For this review, use the dimensioned drawing (mm, ordinates from the lowest corner) and the shaded views. Coordinates: 2 decimals unless noted, no trailing zeros. Write each loop counter-clockwise with the first axis right and the second up, starting at its lowest first coordinate (ties: lowest second). Pieces come first, ordered by that corner, then holes. Notation, with made-up numbers: (8, 73.5) - (25, 73.5) arc R17 cw to (25, 101.5) - close; hole circle Ø10 at (16, 78.5). An arc over 180 degrees is marked (long way). One line per item, written item: value.
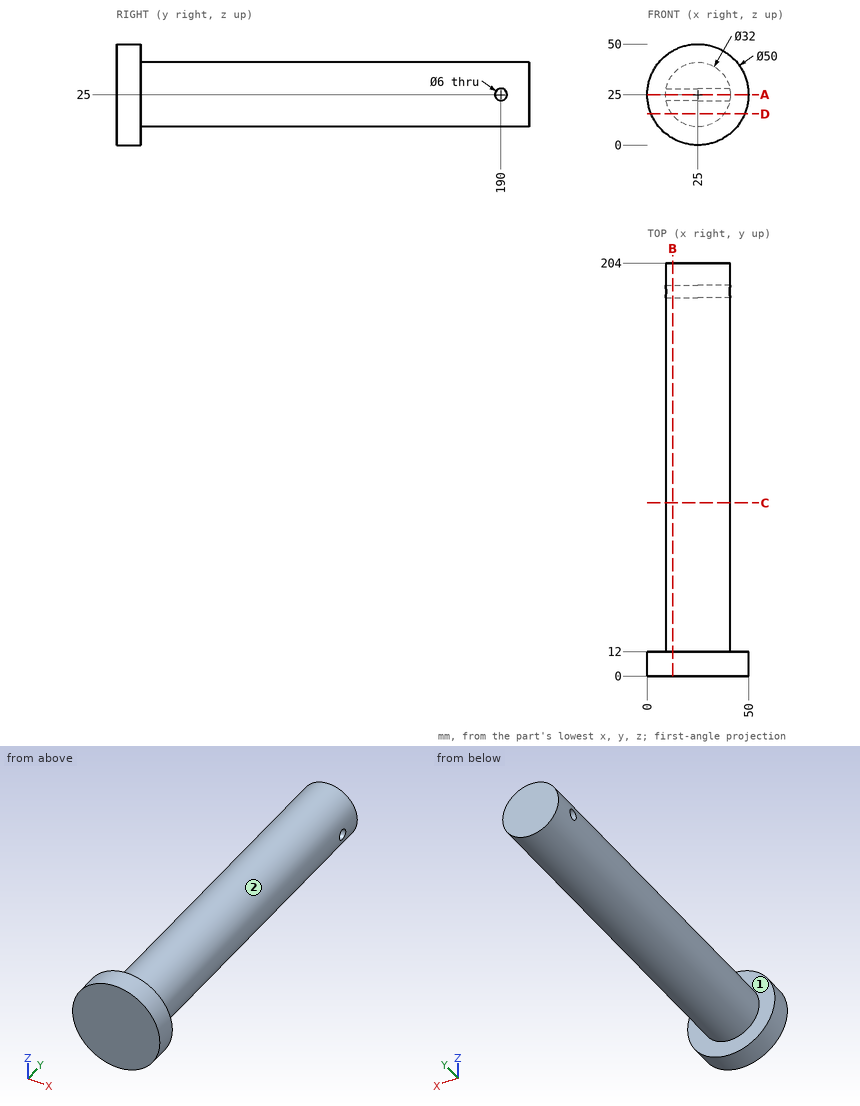
1. Wall thickness on line 1 along Y through (x, z) = (18, 25); line 2 along Y through (x, z) = (22, 43.5); line 3 along Y through (x, z) = (23, 27): over which ranges is each line inside the solid? List them lowest first.
Answer block:
line 1: y = 0 to 187, 193 to 204
line 2: y = 0 to 12
line 3: y = 0 to 187.76, 192.24 to 204
2. Consider section C-C, the plane y = 85.5. Write out the cut boundary in (x, z), then the cut area to 3 significant figures.
Answer block:
outline: circle Ø32 at (25, 25)
area: 804 mm^2
3. Consider section A-A, the plane z = 25. Write out the cut boundary in (x, y), then the cut area to 3 significant figures.
Answer block:
outline: (0, 0) - (50, 0) - (50, 12) - (41, 12) - (41, 187) - (9, 187) - (9, 12) - (0, 12) - close; (9, 193) - (41, 193) - (41, 204) - (9, 204) - close
area: 6,550 mm^2
4. Consider section D-D, the plane z = 15.5. Write out the cut boundary in (x, y).
Answer block:
outline: (1.88, 0) - (48.12, 0) - (48.12, 12) - (37.87, 12) - (37.87, 204) - (12.13, 204) - (12.13, 12) - (1.88, 12) - close
5. Mouldability with a two-part tool opening along X and no side actions: class the marked faces 1 and 2 as released by +X, released by -X, zero draft, split by the parting line, or undercut.
Answer block:
face 1: zero draft
face 2: split by the parting line
6. Insertion check: pin 1 Ø2 at (x, y) = (39, 20.5) entering from +Z; pin 2 Ø12 at (y, z) = (96.5, 39.5) entering from -X; pin 3 Ø8 at (y, z) = (190, 25) entering from -X. Each pin has a flat end and moves straight along its axis. Give the tip position at first contact, or say it passes through.
Answer block:
pin 1: stops at z = 34.33
pin 2: stops at x = 11.44
pin 3: stops at x = 9
7. Consider section B-B, the plane x = 12.5. Write out the cut boundary in (y, z), then the cut area to 3 significant figures.
Answer block:
outline: (0, 3.35) - (12, 3.35) - (12, 15.01) - (204, 15.01) - (204, 34.99) - (12, 34.99) - (12, 46.65) - (0, 46.65) - close; hole circle Ø6 at (190, 25)
area: 4,330 mm^2
